from build123d import *

# Parameters (mm, degrees)
SKETCH_1_W      = 550
SKETCH_1_H      = 400
EXTRUDE_1_DEPTH = 25
FILLET_1_R      = 4
SHELL_1_T       = -2


with BuildPart() as part:
    # 草图1 → 凸台-拉伸1 (new body)
    with BuildSketch(Plane.XY):
        with Locations((275, 200)):
            Rectangle(SKETCH_1_W, SKETCH_1_H)
    extrude(amount=-EXTRUDE_1_DEPTH)

    # 圆角1
    fillet_1_edges = [part.edges().sort_by_distance(p)[0] for p in [
        (275, 400, 0),
        (275, 0, 0),
        (0, 200, 0),
        (0, 400, -12.5),
        (0, 0, -12.5),
    ]]
    fillet(fillet_1_edges, radius=FILLET_1_R)

    # 抽壳1
    shell_1_openings = [part.faces().sort_by_distance(p)[0] for p in [
        (275.008556451, 200, -25),
        (550, 200, -12.507975981),
    ]]
    offset(amount=SHELL_1_T, openings=shell_1_openings, kind=Kind.INTERSECTION)


solid = part.part
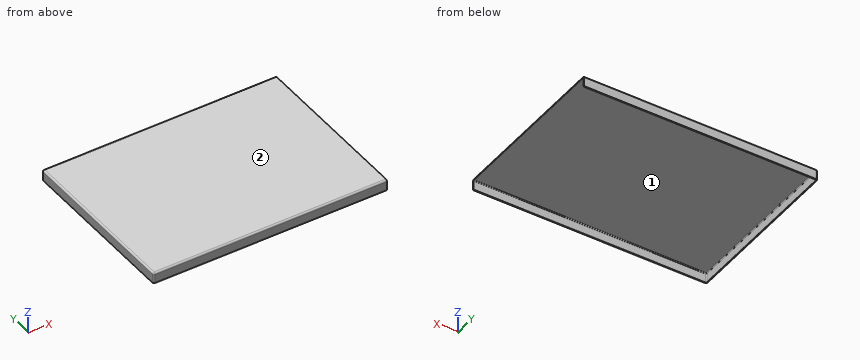
The listing builds one solid part. Answer for the finished solid, in the listing's coordinates (mm). Face numbers are marked on the shaded views. A direction names the side the tool comes from. Give positions to 0.01 mm unless a question says otherwise; leave off trailing zeros. Write each loop counter-clockwise with the first axis right and the second up, starting at its lowest first coordinate (ties: lowest second). Pieces come first, ordered by that corner, then holes. Notation, with made-up numbers: (-14.75, 65) - (20.25, 65) arc R25 ccw to (20.25, 102) - close; hole circle Ø6 at (53, -37). An arc over 180 degrees is marked (long way). Use a Markdown table: item, result.
1. Each of these flat-tipped pins is pushed along its axis until it touches: P1, Ø5, axis at y = 314.5, z = -20.5, coming from the +X side; P2, Ø6, axis at x = 243.5, y = 197, coming from the -Z side. Where does it stop, or does it pass through?
Values follow:
| item | result |
|---|---|
| P1 | stops at x = 2 |
| P2 | stops at z = -2 |
2. Section A-A on z = -8.25 is taken. Write down the section's boundary in (x, y).
Values follow:
| item | result |
|---|---|
| outline | (0, 4) arc R4 ccw to (4, 0) - (550, 0) - (550, 2) - (4, 2) arc R2 cw to (2, 4) - (2, 396) arc R2 cw to (4, 398) - (550, 398) - (550, 400) - (4, 400) arc R4 ccw to (0, 396) - close |
3. Section B-B on y = 85 is taken. Write down the section's boundary in (x, z).
Values follow:
| item | result |
|---|---|
| outline | (0, -25) - (2, -25) - (2, -4) arc R2 cw to (4, -2) - (550, -2) - (550, 0) - (4, 0) arc R4 ccw to (0, -4) - close |
4. A tool of negligible diameter and unlimited length cuts with its end or side. For the marked faces 1 and 2, from which of +Z, -Z, +X, -X, +Y, -Y can it reach the whole face along a straight path? Write none if from no direction.
Values follow:
| item | result |
|---|---|
| face 1 | -Z, +X |
| face 2 | +Z, +X, -X, +Y, -Y |
5. Section C-C on x = 142 is taken. Write down the section's boundary in (y, z).
Values follow:
| item | result |
|---|---|
| outline | (0, -25) - (2, -25) - (2, -4) arc R2 cw to (4, -2) - (396, -2) arc R2 cw to (398, -4) - (398, -25) - (400, -25) - (400, -4) arc R4 ccw to (396, 0) - (4, 0) arc R4 ccw to (0, -4) - close |
6. Find the intervals of material crossed by probe 1 along Y at (x, z) = (261.5, -6.5); probe 2 along Z at (x, y) = (396, 312.5); probe 3 along X at (y, z) = (202.5, -12.75), in increasing order. Write a range as from..to.
Values follow:
| item | result |
|---|---|
| probe 1 | y = 0..2, 398..400 |
| probe 2 | z = -2..0 |
| probe 3 | x = 0..2 |
